Can you work these out from the model? Positions are in its coordinate system, mm. Face numbers are marked on the shaded views. Round coordinates to 2 decimals unless told otherwise and drop trailing zeros. Write each loop counter-clockwise with the first axis right and the second up, starting at its lowest first coordinate (ties: lowest second). Pieces come first, ordered by that corner, then holes.
Q1. If we section it at C-C (z = 8): Give the number of separate pieces and of enclosed holes in the cut face, plus the area to 3 significant figures.
Q2. We'd pull the mould along Y, two halves only. Please class the marked faces 1, 2 and 3: +Y half, -Y half, draft (parallel to the pull), parting line (faces both ways), or undercut.
Q3. If we section it at A-A (x = -18): Please give me the cut outline in (y, z).
Q4. If we section it at B-B (y = -38.5): Please give me the cut outline in (x, z).
Q5. Please list where these lines run through material, in increasing order: line 1 along Y through (x, z) = (-25.5, 3); line 2 along Y through (x, z) = (8, 1); line 3 along X through (y, z) = (1, 4).
Q6. If we section it at D-D (x = 9): Please give me the cut outline in (y, z).
Q7. I'm going to push flat-ended pins straight in: pin 1 Ø1 at (x, z) = (35, 4.5) entering from +Y (3 decimals); pin 2 Ø6.5 at (x, z) = (-2, 7.5) entering from +Y; pin 3 Ø1.5 at (x, z) = (-36, 10.5) entering from -Y. Where does each tip first touch, or does it pass through?
from build123d import *

# Parameters (mm, degrees)
F0_R     = 51.2028826098
F0_R_2   = 11.123942978
F0_R_3   = 12.0781304444
F1_DEPTH = 12.7


with BuildPart() as f1:
    # F0 (on Top) → F1 (new body)
    with BuildSketch(Plane.XY):
        Circle(F0_R)
        with BuildLine():
            ThreePointArc((26.0693728924, -26.4278631657), (-0.7005850014, -44.2258215238), (-28.6329444498, -28.3141508698))
            Line((-28.6329444498, -28.3141508698), (26.0693728924, -26.4278631657))
        make_face(mode=Mode.SUBTRACT)
        with BuildLine():
            add(Edge.make_bspline(
                [(4.1622381729, -4.4216929377), (6.8932937771, 11.1605301499), (0, 11.1605301499), (-6.8932937771, 11.1605301499), (-4.1622381729, -4.4216929377)],
                knots=[1.1634325355, 1.1634325355, 1.1634325355, 3.1415926536, 3.1415926536, 5.1197527717, 5.1197527717, 5.1197527717], degree=2, weights=[1, 0.5494587228, 1, 0.5494587228, 1]))
            Line((4.1622381729, -4.4216929377), (-4.1622381729, -4.4216929377))
        make_face(mode=Mode.SUBTRACT)
        with Locations((-17.6053456962, 21.5351078659)):
            Circle(F0_R_2, mode=Mode.SUBTRACT)
        with Locations((18.2341039181, 20.2775839716)):
            Circle(F0_R_3, mode=Mode.SUBTRACT)
    extrude(amount=F1_DEPTH)


solid = f1.part
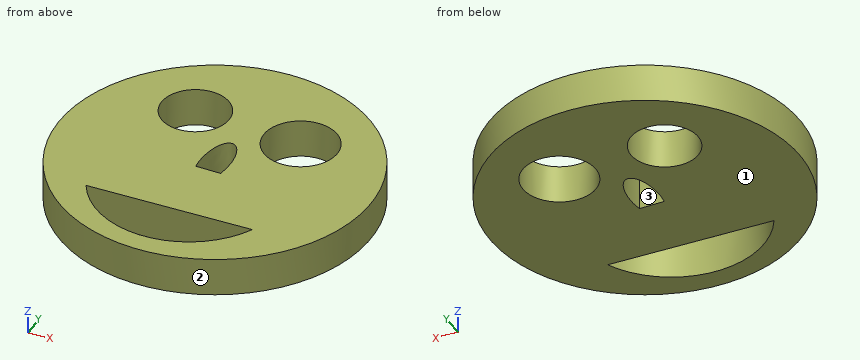
A:
1. separate pieces: 1
1. enclosed holes: 4
1. area: 6,610 mm2
2. face 1: draft
2. face 2: parting line
2. face 3: undercut
3. outline: (-47.93, 0) - (-39.58, 0) - (-39.58, 12.7) - (-47.93, 12.7) - close; (-27.95, 0) - (10.42, 0) - (10.42, 12.7) - (-27.95, 12.7) - close; (32.65, 0) - (47.93, 0) - (47.93, 12.7) - (32.65, 12.7) - close
4. outline: (-33.76, 0) - (-19.62, 0) - (-19.62, 12.7) - (-33.76, 12.7) - close; (16.1, 0) - (33.76, 0) - (33.76, 12.7) - (16.1, 12.7) - close
5. line 1: y = -44.4 to -32.97, -28.21 to 13.7, 29.37 to 44.4
5. line 2: y = -50.57 to -42.65, -27.05 to 13.86, 26.69 to 50.57
5. line 3: x = -51.19 to -4.51, 4.51 to 51.19
6. outline: (-50.41, 0) - (-42.29, 0) - (-42.29, 12.7) - (-50.41, 12.7) - close; (-27.02, 0) - (12.49, 0) - (12.49, 12.7) - (-27.02, 12.7) - close; (28.06, 0) - (50.41, 0) - (50.41, 12.7) - (28.06, 12.7) - close
7. pin 1: stops at y = 37.835
7. pin 2: stops at y = 51.2
7. pin 3: stops at y = -37.14
